Design review of the part built by this model. Coordinates are the model's own, in mm. A direction names the side the tool comes from. Coordinates: 2 decimals unless noted, no trailing zeros. Write each loop counter-clockwise with the first axis right and the second up, starting at its lowest first coordinate (ties: lowest second). Pieces come first, ordered by that corner, then holes. Notation, with made-up numbers: M 72,-20.5 L 91,-20.5 A12 cw 91,-8.5 Z; hole C 88,26.5 d11. An arc over 180 degrees is marked long. Return JSON: item names as keys, results as strings. Group by question number.
```python
from build123d import *

# Parameters (mm, degrees)
SKETCH3_R          = 9.525
CUT_EXTRUDE2_DEPTH = 6.35


with BuildPart() as part:
    # Sketch1 → Revolve1 (revolve)
    with BuildSketch(Plane.XY, mode=Mode.PRIVATE) as revolve1_sk:
        with BuildLine():
            Line((-2.155261469, 2.924738531), (-4.047950886, 4.817427948))
            ThreePointArc((-4.047950886, 4.817427948), (-5.077995018, 5.505681433), (-6.293014916, 5.747363917))
            Line((-6.293014916, 5.747363917), (-25.4, 5.747363917))
            Line((-25.4, 5.747363917), (-25.4, 9.525))
            Line((-25.4, 9.525), (-1.777203317, 9.525))
            Line((-1.777203317, 9.525), (10.922796683, 9.525))
            Line((10.922796683, 9.525), (10.922796683, 4.721941296))
            add(Edge.make_bspline(
                [(10.922796683, 4.721941296), (5.402180861, 3.94606934), (0.277993972, 2.081017838)],
                knots=[0, 0, 0, 1, 1, 1], degree=2))
            ThreePointArc((0.277993972, 2.081017838), (0.141141239, 2.044348258), (0, 2.032))
            ThreePointArc((0, 2.032), (-1.166419102, 2.264015185), (-2.155261469, 2.924738531))
        make_face()
    revolve(revolve1_sk.sketch.rotate(Axis((0, 0, 0), (1, 0, 0)), 90), axis=Axis((0, 0, 0), (1, 0, 0)))

    # Sketch3 → Cut-Extrude2 (cut)
    with BuildSketch(Plane(origin=(10.922796683, 0, 0), x_dir=(0, 0, -1), z_dir=(1, 0, 0))):
        with Locations(Location((0, 0, 0), (0, 0, 180))):
            Circle(SKETCH3_R)
        Polygon((-5.829170486, -4.447932641), (0.937437419, -7.272176044), (6.766607905, -2.824243403), (5.829170486, 4.447932641), (-0.937437419, 7.272176044), (-6.766607905, 2.824243403), align=None, mode=Mode.SUBTRACT)
    extrude(amount=-CUT_EXTRUDE2_DEPTH, mode=Mode.SUBTRACT)


solid = part.part
```
Item 1: Add section A-A (x = -16). Write out the cut boundary in (y, z) (3 decimals).
Item 2: For line 1 (Y direction, x = -19, z = 0) (3 decimals); line 2 (Z direction, x = 3.5, y = -1.25); line 3 (Z direction, x = -2, y = 0.5), list the stretches that pass through material, from the lowest coordinate up.
Item 3: For pin 1 (1 mm diameter, centred on y = 7.5, z = -2, fed in from +X); pin 2 (1.5 mm diameter, centred on x = 3.5, z = -5.5, fed in from +Y); pin 3 (3 mm diameter, centred on x = -4, z = -5.5, fed in from +Y), all flat-tipped, find the tip position at first contact; note any pin that passes through.
Item 4: Machinability: for faces 1 (the cylindrical face through (-15.98, 3.5, -4.56)), 2 (the flat face through (7.8, -0.8, 6.3)), 3 (the flat face through (4.573, 6.2, -2.3)), 4 (the flat face through (7.79, -5.08, -3.81)), 5 (the flat face through (7.8, 0.8, -6.3)), which of the approach directions +Z, -Z, +X, -X, +Y, -Y give a long, thin tool a straight path to every point of the face, cutting with its end or side? Answer none if there is none.
Item 5: The part is to be moulded in two halves that separate along Y. For faces 6 (the flat face through (7.79, -5.84, 2.49)), 7 (the flat face through (7.79, 5.08, 3.81)), 8 (the conical face through (-2.27, 2.7, 1.4)), 9 (the flat face through (10.923, -5, 0)), say which applies: pulls with the +Y half, pulls with the -Y half, needs draft (parallel to the pull), parting line crosses it, or undercut.
Item 6: Add section B-B (z = 8). Write out the cut boundary in (x, y).
Item 7: Add section C-C (x = -3). Write out the cut boundary in (y, z) (3 decimals).
Geometry check:
{
 "1": {"outline": "C 0,0 d19.05; hole C 0,0 d11.495"},
 "2": {"line 1": "-9.525 to -5.747, 5.747 to 9.525", "line 2": "-9.44 to -2.87, 2.87 to 9.44", "line 3": "-9.51 to -2.73, 2.73 to 9.51"},
 "3": {"pin 1": "x = 4.57", "pin 2": "y = 8.26", "pin 3": "y = 8.64"},
 "4": {"face 1": "-X", "face 2": "+Z, +X, -Y", "face 3": "+X", "face 4": "-Z, +X, -Y", "face 5": "-Z, +X, +Y"},
 "5": {"face 6": "pulls with the -Y half", "face 7": "pulls with the +Y half", "face 8": "undercut", "face 9": "needs draft"},
 "6": {"outline": "M -25.4,-5.17 L 4.57,-5.17 L 4.57,5.17 L -25.4,5.17 Z"},
 "7": {"outline": "C 0,0 d19.05; hole C 0,0 d7.539"}
}
